Source: CAD feature listing. Evaluate the final solid. Frame: model axes, mm. A direction names the side the tool comes from. Round coordinates to 2 decimals unless told otherwise and drop trailing zeros. Write each loop counter-clockwise with the first axis right and the second up, starting at its lowest first coordinate (ties: lowest second). Pieces come first, ordered by that corner, then holes. Notation, with made-up numbers: (13, 9.25) -> (38, 9.25) arc R32 cw to (38, 42.25) -> close; hole circle Ø11 at (18, -39.5). An arc over 180 degrees is marked (long way). Put each result on its own line as item: value.
```python
from build123d import *

# Parameters (mm, degrees)
SKETCH3_W               = 4
SKETCH3_H               = 10
CUT_EXTRUDE2_DEPTH      = 11.5
CUT_EXTRUDE3_DEPTH      = 30.711019541
CUT_EXTRUDE3_DEPTH_BACK = 30.711019541
BOSS_EXTRUDE1_DEPTH     = 1.5
CUT_EXTRUDE4_DEPTH      = 30.711019541
CUT_EXTRUDE4_DEPTH_BACK = 30.711019541
SKETCH5_R               = 1.5


with BuildPart() as part:
    # Sketch1 → Revolve1 (revolve)
    with BuildSketch(Plane(origin=(0, 0, 0), x_dir=(0, 0, -1), z_dir=(1, 0, 0))):
        with BuildLine():
            Line((0, 0), (0, 28))
            Line((0, 28), (5.5, 28))
            add(Edge.make_bspline(
                [(5.5, 28), (8.278370843, 12.243075952), (6, 0)],
                knots=[0, 0, 0, 1, 1, 1], degree=2))
            Line((6, 0), (0, 0))
        make_face()
    revolve(axis=Axis((0, 0, 0), (0, 1, 0)))

    # Sketch3 → Cut-Extrude2 (cut, symmetric)
    with BuildSketch(Plane.XY):
        with Locations((0, 23)):
            Rectangle(SKETCH3_W, SKETCH3_H)
    extrude(amount=CUT_EXTRUDE2_DEPTH, both=True, mode=Mode.SUBTRACT)

    # Sketch4 → Cut-Extrude3 (cut, two sides: drawn at the far end of the back side and taken through both)
    with BuildSketch(Plane(origin=(0, 0, 0), x_dir=(0, 0, -1), z_dir=(1, 0, 0)).offset(-CUT_EXTRUDE3_DEPTH_BACK)):
        Polygon((-6.781758395, 28), (-6.480142509, 18), (0.363394388, 28), align=None)
    extrude(amount=CUT_EXTRUDE3_DEPTH + CUT_EXTRUDE3_DEPTH_BACK, mode=Mode.SUBTRACT)

    # Sketch6 → Boss-Extrude1 (add, symmetric)
    with BuildSketch(Plane(origin=(0, 0, 0), x_dir=(0, 0, -1), z_dir=(1, 0, 0))):
        Polygon((-6, 0), (-6, -6), (0, -10), (6, -10), (6, 0), align=None)
    extrude(amount=BOSS_EXTRUDE1_DEPTH, both=True)

    # Sketch5 → Cut-Extrude4 (cut, two sides: drawn at the far end of the back side and taken through both)
    with BuildSketch(Plane(origin=(0, 0, 0), x_dir=(0, 0, -1), z_dir=(1, 0, 0)).offset(-CUT_EXTRUDE4_DEPTH_BACK)):
        with Locations((2.5, 23)):
            Circle(SKETCH5_R)
        with Locations(Location((2.5, -5, 0), (0, 0, 180))):
            Circle(SKETCH5_R)
    extrude(amount=CUT_EXTRUDE4_DEPTH + CUT_EXTRUDE4_DEPTH_BACK, mode=Mode.SUBTRACT)


solid = part.part
```
Q1. Draft query along Z for faces 1 (the flat face through (1.5, -5, 0)), 2 (the cylindrical face through (0, -5, -1)), 3 (the cylindrical face through (-3.7, 22.1, -1.3)), 4 (the flat face through (0, -5, -6)). Return one class per face: +Z half, -Z half, draft (parallel to the pull), parting line (faces both ways), or undercut.
Ans:
face 1: draft
face 2: undercut
face 3: undercut
face 4: -Z half
Q2. Material intervals for line 1 (Y direction, x = 0.05, z = -2.5); line 2 (Y direction, x = 4.45, z = -2.5); line 3 (Z direction, x = -3.1, y = 23), sorted ascending. Write a range as [from, to].
Ans:
line 1: y = [-10, -6.5], [-3.5, 18]
line 2: y = [0, 21.5], [24.5, 28]
line 3: z = [-5.45, -4], [-1, 3.06]
Q3. Pin query (flat end, axial travel): pin 1 (5 mm diameter, centred on x = 4, y = 20.5, fed in from -Z); pin 2 (4 mm diameter, centred on y = 0.5, z = 2.5, fed in from +X); pin 3 (4 mm diameter, centred on y = 14, z = -4.5, fed in from -X); pin 4 (4 mm diameter, centred on x = 2, z = 0, fed in from +Y). Return the tip coordinate at first contact, or that it passes through.
Ans:
pin 1: stops at z = -6.39
pin 2: stops at x = 6.23
pin 3: stops at x = -6.53
pin 4: stops at y = 28
Q4. Cut plane A-A on y = -5. Output: boundary loops of the cut face in (x, z).
Ans:
outline: (-1.5, -6) -> (1.5, -6) -> (1.5, -4) -> (-1.5, -4) -> close; (-1.5, -1) -> (1.5, -1) -> (1.5, 6) -> (-1.5, 6) -> close
Q5. Cut plane B-B on z = -2.5. Give the number of separate pieces and of enclosed holes in the cut face, and give its area (3 significant figures).
Ans:
separate pieces: 4
enclosed holes: 0
area: 299 mm^2
Q6. Reachability of faces 5 (the flat face through (-3, 0, 0)), 6 (the flat face through (0, -3, 6)), 7 (the flat face through (3, 0, 0)), 8 (the flat face through (0, 18, 0)) from +Z, -Z, +X, -X, +Y, -Y: full face, straight path, thin tool, end or side. Return the list, or none.
Ans:
face 5: +Z, -Z, -X, -Y
face 6: +Z, +X, -X, -Y
face 7: +Z, -Z, +X, -Y
face 8: +Z, -Z, +Y
